Could you check a few things on this model? Use its own coordinates, in mm. A direction names the side the tool comes from. Give positions to 0.01 mm unless a question says otherwise; leave off trailing zeros. Loops run counter-clockwise (first coordinate to the right, second up) from the corner with the lowest first, then second, coordinate; pieces in that order, holes last. Notation, with made-up numbers: (70, 3) - (88, 3) arc R21 cw to (88, 34) - close; hole circle Ø10 at (54, 83.5). An arc over 180 degrees is marked (long way). Answer in a Markdown table with one row per item. Add a question column.
```python
from build123d import *

# Parameters (mm, degrees)
F0_R          = 54.948812
F1_DEPTH      = 50.8
F1_DEPTH_BACK = 25.4
F2_T          = -7.62
F4_DEPTH      = 68.58


with BuildPart() as f1:
    # F0 (on Top) → F1 (new body, two sides)
    with BuildSketch(Plane.XY) as f1_sk:
        Circle(F0_R)
    extrude(amount=F1_DEPTH)
    extrude(f1_sk.sketch, amount=-F1_DEPTH_BACK)

    # F2
    f2_openings = [f1.faces().sort_by_distance(p)[0] for p in [
        (0, 0, 50.8),
    ]]
    offset(amount=F2_T, openings=f2_openings)

    # F3 (on face) → F4 (join)
    with BuildSketch(Plane.XY.offset(-17.78)):
        Polygon((29.444208, -16.999622), (29.444208, 16.999622), (0, 33.999243), (-29.444208, 16.999622), (-29.444208, -16.999622), (0, -33.999243), align=None)
    extrude(amount=F4_DEPTH)


solid = f1.part
```
(1) We'd pull the mould along X, two halves only. Please class faces 1 (the flat face through (24, 41, 50.8)), 2 (the cylindrical face through (-11.912, -53.642, 13.233)), 3 (the flat face through (29.444, 0, 16)): pulls with the +X half, pulls with the -X half, needs draft (parallel to the pull), parting line crosses it, or undercut.
(2) I want a section at B-B on y = 0. Please give me the cut outline in (x, z).
(3) Please list where these lines run through material, in increasing order: line 1 (Y direction, x = 0, z = 28); line 2 (X direction, y = 1, z = 31.5); line 3 (Y direction, x = -6, z = -10).
(4) On a 3-axis mill with a long thin cutter (end or side, diameter ignored), from which of +Z, -Z, +X, -X, +Y, -Y can I reach the whole of each face in a straight line? I mean faces 4 (the flat face through (-29.444, 0, 16)), 5 (the flat face through (-1, 1, -25.4)). Say none if no direction works.
(5) I want a section at A-A on z = 4. Please give me the cut outline in (x, y), then the cut area to 3 significant figures.
(6) I want a section at D-D on y = -42.5. Please give me the cut outline in (x, z).
(7) I want a section at C-C on x = 44. Please give me the cut outline in (y, z), then the cut area to 3 significant figures.
(8) For pin 1 Ø4 at (y, z) = (37, 14) entering from -X; pin 2 Ø8 at (y, z) = (-15, -6) entering from -X; pin 3 Ø8 at (y, z) = (-10, 20) entering from -X, each with a flat end and sliding along its axis, tell me the tip position at first contact or that it passes through.
Reported:
| question | item | result |
|---|---|---|
| 1 | face 1 | needs draft |
| 1 | face 2 | parting line crosses it |
| 1 | face 3 | undercut |
| 2 | outline | (-54.95, -25.4) - (54.95, -25.4) - (54.95, 50.8) - (47.33, 50.8) - (47.33, -17.78) - (29.44, -17.78) - (29.44, 50.8) - (-29.44, 50.8) - (-29.44, -17.78) - (-47.33, -17.78) - (-47.33, 50.8) - (-54.95, 50.8) - close |
| 3 | line 1 | -54.95 to -47.33, -34 to 34, 47.33 to 54.95 |
| 3 | line 2 | -54.94 to -47.32, -29.44 to 29.44, 47.32 to 54.94 |
| 3 | line 3 | -54.62 to -46.95, -30.54 to 30.54, 46.95 to 54.62 |
| 4 | face 4 | +Z |
| 4 | face 5 | -Z, +X, -X, +Y, -Y |
| 5 | outline | circle Ø109.9 at (0, 0); (-29.44, -17) - (0, -34) - (29.44, -17) - (29.44, 17) - (0, 34) - (-29.44, 17) - close; hole circle Ø94.66 at (0, 0) |
| 5 | area | 5,450 mm² |
| 6 | outline | (-34.83, -25.4) - (34.83, -25.4) - (34.83, 50.8) - (20.83, 50.8) - (20.83, -17.78) - (-20.83, -17.78) - (-20.83, 50.8) - (-34.83, 50.8) - close |
| 7 | outline | (-32.91, -25.4) - (32.91, -25.4) - (32.91, 50.8) - (17.44, 50.8) - (17.44, -17.78) - (-17.44, -17.78) - (-17.44, 50.8) - (-32.91, 50.8) - close |
| 7 | area | 2,620 mm² |
| 8 | pin 1 | x = -42.36 |
| 8 | pin 2 | x = -53.84 |
| 8 | pin 3 | x = -54.62 |
